```python
from build123d import *

# Parameters (mm, degrees)
SKETCH1_W           = 150
SKETCH1_H           = 250
BOSS_EXTRUDE1_DEPTH = 180
SHELL1_T            = -3
SKETCH2_W           = 150
SKETCH2_H           = 3
BOSS_EXTRUDE2_DEPTH = 180
SKETCH3_R           = 15
CUT_EXTRUDE1_DEPTH  = 10
FILLET1_R           = 2
SKETCH9_R           = 13
CUT_EXTRUDE2_DEPTH  = 15
SKETCH9_3_R         = 15
SKETCH9_3_R_2       = 13
BOSS_EXTRUDE3_DEPTH = 40


with BuildPart() as part:
    # Sketch1 → Boss-Extrude1 (new body)
    with BuildSketch(Plane.XY):
        with Locations((75, -125)):
            Rectangle(SKETCH1_W, SKETCH1_H)
    extrude(amount=BOSS_EXTRUDE1_DEPTH)

    # Shell1
    shell1_openings = [part.faces().sort_by_distance(p)[0] for p in [
        (75, 0, 90),
    ]]
    offset(amount=SHELL1_T, openings=shell1_openings, kind=Kind.INTERSECTION)

    # Sketch2 → Boss-Extrude2 (add)
    with BuildSketch(Plane.XY):
        with Locations((75, -1.5)):
            Rectangle(SKETCH2_W, SKETCH2_H)
    extrude(amount=BOSS_EXTRUDE2_DEPTH)

    # Sketch3 → Cut-Extrude1 (cut)
    with BuildSketch(Plane(origin=(0, 0, 0), x_dir=(1, 0, 0), z_dir=(0, 1, 0))):
        with Locations((30, -120)):
            Circle(SKETCH3_R)
    extrude(amount=-CUT_EXTRUDE1_DEPTH, mode=Mode.SUBTRACT)

    # Fillet1
    fillet1_edges = [part.edges().sort_by_distance(p)[0] for p in [
        (150, -125, 180),
        (75, 0, 180),
        (15, 0, 120),
        (0, -125, 180),
        (75, 0, 0),
        (150, -125, 0),
        (0, -125, 0),
        (0, 0, 90),
        (150, 0, 90),
        (150, -250, 90),
        (0, -250, 90),
        (75, -250, 180),
    ]]
    fillet(fillet1_edges, radius=FILLET1_R)

    # Sketch9 → Cut-Extrude2 (cut)
    with BuildSketch(Plane(origin=(0, 0, 0), x_dir=(-1, 0, 0), z_dir=(0, 0, -1))):
        with Locations((-70, -235)):
            Circle(SKETCH9_R)
    extrude(amount=-CUT_EXTRUDE2_DEPTH, mode=Mode.SUBTRACT)

    # Sketch9_3 → Boss-Extrude3 (add)
    with BuildSketch(Plane(origin=(0, 0, 0), x_dir=(-1, 0, 0), z_dir=(0, 0, -1))):
        with Locations((-70, -235)):
            Circle(SKETCH9_3_R)
        with Locations((-70, -235)):
            Circle(SKETCH9_3_R_2, mode=Mode.SUBTRACT)
    extrude(amount=BOSS_EXTRUDE3_DEPTH)


solid = part.part
```
Model file for the job. Use its own axes, mm. A direction names the side the tool comes from. Coordinates: 2 decimals unless noted, no trailing zeros. Order: outer loops, then holes, each group sorted by start corner. A loop starts at its lowest first (then second) coordinate and runs counter-clockwise, first axis right, second up. Notation, with made-up numbers: (51, -39.5) -> (84, -39.5) arc R37 cw to (84, -3.5) -> close; hole circle Ø1 at (52.25, 11.5). An arc over 180 degrees is marked (long way). Answer as a JSON object with one key per item and string values. Group by question number.
1) Cut at C-C, the plane y = -50. Write the cut outline in (x, z), then the cut area to 3 significant figures.
2) Drill centre lines: L1, parallel to Z at x = 42, y = -44; L2, parallel to X at y = -2, z = 120; L3, parallel to Y at x = 76.5, z = 112.5. Where is each one in solid material? Low to high.
3) Cut at A-A, the plane z = 10.5. Write the cut outline in (x, y).
4) Pull direction X, two halves, no side cores. Call faces 4 (the face through (74, -250, 88)), 5 (the face through (150, -127, 89)), 6 (the face through (28.047, -2.493, 105.128)): +X half, -X half, draft (parallel to the pull), parting line (faces both ways), or undercut.
5) Cut at D-D, the plane x = 30. Write the cut outline in (y, z).
6) Cut at B-B, the plane x = 137.5. Write the cut outline in (y, z), then the cut area to 3 significant figures.
7) Flat gauge pins, fed straight in: pin 1 (24 mm diameter, centred on x = 30, z = 120, fed in from +Y); pin 2 (3 mm diameter, centred on x = 66.5, y = -193.5, fed in from -Z). Where does each tip first touch, or does it go through?
8) Which spindle directions (+Z, -Z, +X, -X, +Y, -Y) get a long thin tool onto all of the face, cutting with end or side? Do faces 1 (the face through (73.252, -249.643, -19.72)), 2 (the face through (147, -127, 89)), 3 (the face through (70.1, -221.6, -40)). Say none if no direction does.
Check values:
{
 "1": {"outline": "(0, 2) arc R2 ccw to (2, 0) -> (148, 0) arc R2 ccw to (150, 2) -> (150, 178) arc R2 ccw to (148, 180) -> (2, 180) arc R2 ccw to (0, 178) -> close; hole (3, 3) -> (147, 3) -> (147, 177) -> (3, 177) -> close", "area": "1,940 mm²"},
 "2": {"L1": "z = 0 to 3, 177 to 180", "L2": "x = 0 to 15, 45 to 150", "L3": "y = -250 to -247, -3 to 0"},
 "3": {"outline": "(0, -248) arc R2 ccw to (2, -250) -> (148, -250) arc R2 ccw to (150, -248) -> (150, -2) arc R2 ccw to (148, 0) -> (2, 0) arc R2 ccw to (0, -2) -> close; hole (3, -247) -> (65, -247) arc R13 ccw to (75, -247) -> (147, -247) -> (147, -3) -> (3, -3) -> close"},
 "4": {"face 4": "draft", "face 5": "+X half", "face 6": "undercut"},
 "5": {"outline": "(-250, 0) -> (-2, 0) arc R2 ccw to (0, 2) -> (0, 103) arc R2 ccw to (-2, 105) -> (-3, 105) -> (-3, 3) -> (-247, 3) -> (-247, 177) -> (-3, 177) -> (-3, 135) -> (-2, 135) arc R2 ccw to (0, 137) -> (0, 178) arc R2 ccw to (-2, 180) -> (-248, 180) arc R2 ccw to (-250, 178) -> close"},
 "6": {"outline": "(-250, 0) -> (-2, 0) arc R2 ccw to (0, 2) -> (0, 178) arc R2 ccw to (-2, 180) -> (-248, 180) arc R2 ccw to (-250, 178) -> close; hole (-247, 3) -> (-3, 3) -> (-3, 177) -> (-247, 177) -> close", "area": "2,540 mm²"},
 "7": {"pin 1": "stops at y = -247", "pin 2": "stops at z = 0"},
 "8": {"face 1": "-Z", "face 2": "none", "face 3": "-Z, +X, -X, +Y, -Y"}
}
